```python
from build123d import *

# Parameters (mm, degrees)
FILLET1_R           = 0.1
SKETCH2_R           = 0.25
BOSS_EXTRUDE1_DEPTH = 10
SKETCH3_R           = 0.25
BOSS_EXTRUDE2_DEPTH = 7


with BuildPart() as part:
    # Sketch1 one side → Revolve6 (revolve)
    with BuildSketch(Plane.XY):
        with BuildLine():
            Line((0, 0), (2, 0))
            Line((2, 0), (2, 0.8))
            Line((2, 0.8), (1.6, 0.8))
            Line((1.6, 0.8), (1.6, 4.4))
            ThreePointArc((1.6, 4.4), (1.13137085, 5.53137085), (0, 6))
            Line((0, 6), (0, 0))
        make_face()
    revolve(axis=Axis((0, 8.598320721, 0), (0, -1, 0)))

    # Fillet1
    fillet1_edges = [part.edges().sort_by_distance(p)[0] for p in [
        (-2, 0, 0),
        (-2, 0.8, 0),
    ]]
    fillet(fillet1_edges, radius=FILLET1_R)

    # Sketch2 → Boss-Extrude1 (add)
    with BuildSketch(Plane.XZ):
        with Locations((-1.27, 0)):
            Circle(SKETCH2_R)
    extrude(amount=BOSS_EXTRUDE1_DEPTH)

    # Sketch3 → Boss-Extrude2 (add)
    with BuildSketch(Plane.XZ):
        with Locations((1.27, 0)):
            Circle(SKETCH3_R)
    extrude(amount=BOSS_EXTRUDE2_DEPTH)


solid = part.part
```
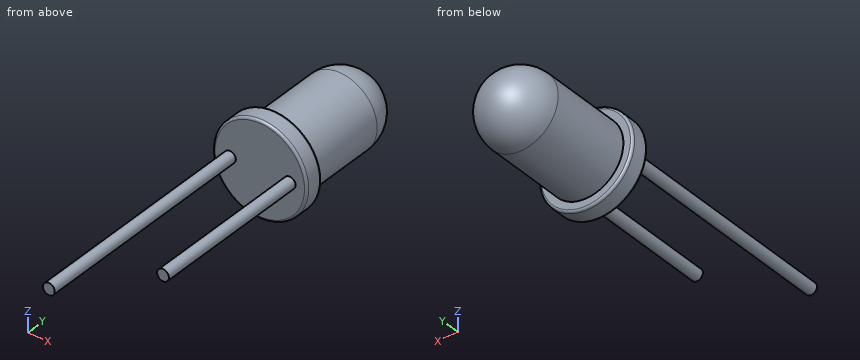
Input: part model. Units: mm. Frame: model coordinates. Coordinates: 2 decimals unless noted, no trailing zeros. Loops run counter-clockwise (first coordinate to the right, second up) from the corner with the lowest first, then second, coordinate; pieces in that order, holes last. Notation, with made-up numbers: (69.5, 75.5) -> (82.5, 75.5) arc R23 ccw to (82.5, 84.5) -> close; hole circle Ø5 at (-33.5, 24.25). An arc over 180 degrees is marked (long way). Use a Markdown table: item, result.
1) Cut plane C-C (z = 0). Return the cut outline in (x, y).
Results found:
| item | result |
|---|---|
| outline | (-2, 0.1) arc R0.1 ccw to (-1.9, 0) -> (-1.52, 0) -> (-1.52, -10) -> (-1.02, -10) -> (-1.02, 0) -> (1.02, 0) -> (1.02, -7) -> (1.52, -7) -> (1.52, 0) -> (1.9, 0) arc R0.1 ccw to (2, 0.1) -> (2, 0.7) arc R0.1 ccw to (1.9, 0.8) -> (1.6, 0.8) -> (1.6, 4.4) arc R1.6 ccw to (-1.6, 4.4) -> (-1.6, 0.8) -> (-1.9, 0.8) arc R0.1 ccw to (-2, 0.7) -> close |
2) Cut plane B-B (x = 0). Return the cut outline in (y, z), then the cut area to 3 significant figures.
Results found:
| item | result |
|---|---|
| outline | (0, -1.9) arc R0.1 ccw to (0.1, -2) -> (0.7, -2) arc R0.1 ccw to (0.8, -1.9) -> (0.8, -1.6) -> (4.4, -1.6) arc R1.6 ccw to (4.4, 1.6) -> (0.8, 1.6) -> (0.8, 1.9) arc R0.1 ccw to (0.7, 2) -> (0.1, 2) arc R0.1 ccw to (0, 1.9) -> close |
| area | 18.7 mm2 |
3) Material intervals for line 1 along Z through (x, y) = (-0.1, 3.25); line 2 along Y through (x, z) = (-1.65, 0.7); line 3 along X through (y, z) = (4, -1.25), sorted ascending. Write a range as from..to.
Results found:
| item | result |
|---|---|
| line 1 | z = -1.6..1.6 |
| line 2 | y = 0..0.8 |
| line 3 | x = -1..1 |
4) Cut plane A-A (y = -3.5). Return the cut outline in (x, z).
Results found:
| item | result |
|---|---|
| outline | circle Ø0.5 at (-1.27, 0); circle Ø0.5 at (1.27, 0) |
5) Contact query for flat-ended pins moving along their axis: pin 1 (1.9 mm diameter, centred on x = -1, z = 1, fed in from +Y); pin 2 (0.6 mm diameter, centred on x = 1, z = 0, fed in from -Y). Output: stop coordinate, or through.
Results found:
| item | result |
|---|---|
| pin 1 | stops at y = 5.93 |
| pin 2 | stops at y = -7 |
6) Cut plane D-D (y = 1.75). Return the cut outline in (x, z).
Results found:
| item | result |
|---|---|
| outline | circle Ø3.2 at (0, 0) |
